Autodesk Inventor part; units mm, degrees
ref_plane "YZ Plane" through (0, 0, 0) normal (1, 0, 0) x (0, 1, 0)
ref_plane "XZ Plane" through (0, 0, 0) normal (0, 1, 0) x (-1, 0, 0)
ref_plane "XY Plane" through (0, 0, 0) normal (0, 0, 1) x (1, 0, 0)
sketch "草图1" plane through (0, 0, 0) normal (0, 1, 0) x (-1, 0, 0)
  line L0 (12.4499, -13) -> (-12.4499, -13)
  line L1 (12.4499, 13) -> (-12.4499, 13)
  line L2 (21.8859, 0) -> (-29.1909, 0)
  line L3 (17.5499, 4) -> (14, 4)
  line L4 (14, 4) -> (14, -4)
  line L5 (14, -4) -> (17.5499, -4)
  line L6 (22, 4) -> (14, -4) construction
  line L7 (14, 4) -> (22, -4) construction
  line L8 (-17.5499, 4) -> (-14, 4)
  line L9 (-14, 4) -> (-14, -4)
  line L10 (-14, -4) -> (-17.5499, -4)
  line L11 (-22, 4) -> (-14, -4) construction
  line L12 (-14, 4) -> (-22, -4) construction
  arc A0 (12.4499, -13) -> (17.5499, -4) centre (0, 0) ccw
  arc A1 (17.5499, 4) -> (12.4499, 13) centre (0, 0) ccw
  arc A2 (-12.4499, 13) -> (-17.5499, 4) centre (0, 0) ccw
  arc A3 (-17.5499, -4) -> (-12.4499, -13) centre (0, 0) ccw
  point P0 (18, 0)
  point P1 (-18, 0)
  dimension "d1" = 26
  dimension "d2" = 8
  dimension "d3" = 8
  dimension "d4" = 8
  dimension "d5" = 8
extrude "拉伸1" add sketch "草图1" along normal blind 4
sketch "草图2" plane through (0, 4, 0) normal (0, 1, 0) x (1, 0, 0)
  arc A0 (17.5499, 4) -> (12.4499, 13) centre (0, 0) ccw
  circle A1 centre (0, 0) radius 9.5
  dimension "d8" = 19
extrude "拉伸2" add sketch "草图2" along normal blind 10
sketch "草图3" plane through (0, 14, 0) normal (0, 1, 0) x (1, 0, 0)
  circle A0 centre (0, 0) radius 9.5
  circle A1 centre (0, 0) radius 13
  dimension "d11" = 26
extrude "拉伸3" add sketch "草图3" along normal blind 5 contours A0 | A1
sketch "草图4" plane through (0, 19, 0) normal (0, 1, 0) x (1, 0, 0)
  circle A0 centre (0, 0) radius 13
  line L0 (-22.4415, 0) -> (25.3714, 0)
  line L1 (-6.0622, 11.5) -> (6.0622, 11.5)
  line L2 (-6.0622, -11.5) -> (6.0622, -11.5)
  dimension "d14" = 23
extrude "拉伸4" cut sketch "草图4" against normal blind 5 contours L1 A0 | A0 L2
sketch "草图5" plane through (-6.0622, 19, 11.5) normal (0, 0, 1) x (1, 0, 0)
  line L0 (0, 0) -> (12.1244, 0)
  line L1 (15.5622, -5) -> (-3.4378, -5)
  line L2 (-3.4378, -15) -> (15.5622, -15)
  line L3 (6.0622, -19) -> (6.0622, 3.3866)
  line L4 (2.0622, -8) -> (2.0622, -5)
  line L5 (2.0622, -5) -> (10.0622, -5)
  line L6 (10.0622, -5) -> (10.0622, -8)
  line L7 (10.0622, -8) -> (2.0622, -5) construction
  line L8 (2.0622, -8) -> (10.0622, -5) construction
  arc A0 (2.0622, -8) -> (10.0622, -8) centre (6.0622, -8) ccw
  point P0 (6.0622, -6.5)
  dimension "d17" = 8
  dimension "d18" = 3
extrude "拉伸5" add sketch "草图5" against normal blind 5
sketch "草图6" plane through (6.0622, 19, -11.5) normal (0, 0, -1) x (-1, 0, 0)
  line L0 (10.0622, -8) -> (10.0622, -5)
  line L1 (2.0622, -5) -> (10.0622, -5)
  line L2 (2.0622, -5) -> (2.0622, -8)
  line L3 (-3.4378, -15) -> (15.5622, -15)
  spline S0 degree 2 poles (2.0622, -8) (2.0622, -12) (6.0622, -12) (10.0622, -12) (10.0622, -8) knots 0 0 0 0.5 0.5 1 1 1 weights 1 0.707107 1 0.707107 1
  point P0 (6.0622, -19)
extrude "拉伸6" add sketch "草图6" against normal blind 5
sketch "草图7" plane through (-6.0622, 19, 11.5) normal (0, 0, 1) x (1, 0, 0)
  arc A0 (2.0622, -8) -> (10.0622, -8) centre (6.0622, -8) ccw
  circle A1 centre (6.0622, -8) radius 2
  point P0 (6.0622, -19)
  dimension "d23" = 4
extrude "拉伸7" cut sketch "草图7" against normal blind 30
sketch "草图8" plane through (0, 19, 0) normal (0, 1, 0) x (1, 0, 0)
  arc A0 (6.0622, -11.5) -> (6.0622, 11.5) centre (0, 0) ccw
  circle A1 centre (0, 0) radius 7
  dimension "d26" = 14
extrude "拉伸8" cut sketch "草图8" against normal blind 13
sketch "草图9" plane through (0, 0, 0) normal (0, -1, 0) x (1, 0, 0)
  arc A0 (-17.5499, -4) -> (-12.4499, -13) centre (0, 0) ccw
  circle A1 centre (0, 0) radius 3
  dimension "d29" = 6
extrude "拉伸9" cut sketch "草图9" against normal blind 13
Could you check a few things on this model? Use its own coordinates, in mm. A direction names the side the tool comes from. Coordinates: 2 decimals unless noted, no trailing zeros. Loops run counter-clockwise (first coordinate to the right, second up) from the corner with the lowest first, then second, coordinate; pieces in that order, holes last. Notation, with made-up numbers: (33.25, 65) -> (39.25, 65) arc R17 cw to (39.25, 97) -> close; hole circle Ø8 at (72, 17). An arc over 180 degrees is marked (long way). Answer in a Markdown table with one row per item.
(1) If I drill on probe 1 along Y at (x, z) = (8.5, 4.75); probe 2 along Z at (x, y) = (0, 4.2); probe 3 along Y at (x, z) = (0, -10), over which ranges is the centre line in solid material (lowest first)?
Results found:
| item | result |
|---|---|
| probe 1 | y = 0 to 4, 14 to 19 |
| probe 2 | z = -9.5 to -3, 3 to 9.5 |
| probe 3 | y = 0 to 4, 7 to 9, 13 to 19 |
(2) Imagine slicing it at D-D (z = 9). List the corners of the cut face in (x, y) for me.
Results found:
| item | result |
|---|---|
| outline | (-15.59, 0) -> (15.59, 0) -> (15.59, 4) -> (3.04, 4) -> (3.04, 8.4) arc R4 ccw to (4, 11) -> (4, 14) -> (9.38, 14) -> (9.38, 19) -> (-9.38, 19) -> (-9.38, 14) -> (-4, 14) -> (-4, 11) arc R4 ccw to (-3.04, 8.4) -> (-3.04, 4) -> (-15.59, 4) -> close; hole circle Ø4 at (0, 11) |
(3) Imagine slicing it at C-C (x = 0). Give the number of separate pieces and of enclosed holes in the cut face, plus the area to 3 significant figures.
Results found:
| item | result |
|---|---|
| separate pieces | 4 |
| enclosed holes | 0 |
| area | 183 mm^2 |
(4) Will these pins go through, and if not, where does the flat tip stop? pin 1 Ø1.1 at (x, y) = (-16.5, 1) entering from +Z; pin 2 Ø2 at (y, z) = (4, -2.5) entering from -X; pin 3 Ø6 at (x, y) = (1, 12.5) entering from -Z.
Results found:
| item | result |
|---|---|
| pin 1 | stops at z = 8.34 |
| pin 2 | stops at x = -14 |
| pin 3 | stops at z = -11.5 |
(5) For faces 1 (the face through (0, 14, -11.5)), 2 (the face through (-16, 2, 4)), 3 (the face through (-13, 16, 0)), 4 (the face through (0, 7, 10)), which set-ups out of +Z, -Z, +X, -X, +Y, -Y let a thin tool reach every point of the face, with its end or its side?
Results found:
| item | result |
|---|---|
| face 1 | -Z, +X, -X, +Y |
| face 2 | -X, +Y, -Y |
| face 3 | -X, +Y |
| face 4 | +Z |
(6) Imagine slicing it at B-B (y = 16). List the corners of the cut face in (x, z) for me, plus the area to 3 significant figures.
Results found:
| item | result |
|---|---|
| outline | (-6.06, -11.5) -> (6.06, -11.5) arc R13 ccw to (6.06, 11.5) -> (-6.06, 11.5) arc R13 ccw to start; hole circle Ø14 at (0, 0) |
| area | 352 mm^2 |
(7) Imagine slicing it at A-A (z = 0). List the corners of the cut face in (x, y) for me.
Results found:
| item | result |
|---|---|
| outline | (-14, 0) -> (-3, 0) -> (-3, 6) -> (-7, 6) -> (-7, 19) -> (-13, 19) -> (-13, 14) -> (-9.5, 14) -> (-9.5, 4) -> (-14, 4) -> close; (3, 0) -> (14, 0) -> (14, 4) -> (9.5, 4) -> (9.5, 14) -> (13, 14) -> (13, 19) -> (7, 19) -> (7, 6) -> (3, 6) -> close |
(8) Thinking about a two-plate mould opening in Y: for faces 5 (the face through (-15.7, 2, -8.8)), 6 (the face through (-4, 4, 9)), 7 (the face through (1, 6, 3)), 8 (the face through (-4, 0, 0)), which applies, released by +Y, released by -Y, zero draft, split by the parting line, or undercut?
Results found:
| item | result |
|---|---|
| face 5 | zero draft |
| face 6 | undercut |
| face 7 | released by +Y |
| face 8 | released by -Y |
